```python
from build123d import *

# Parameters (mm, degrees)
ESBO_O1_R                = 12.5
RESSALTO_EXTRUS_O1_DEPTH = 30
ESBO_O2_R                = 8
CORTE_EXTRUS_O1_DEPTH    = 15
ESBO_O3_W                = 3
ESBO_O3_H                = 5
CORTE_EXTRUS_O2_DEPTH    = 6.5


with BuildPart() as part:
    # Esboço1 → Ressalto-extrusão1 (new body)
    with BuildSketch(Plane(origin=(0, 0, 0), x_dir=(1, 0, 0), z_dir=(0, 1, 0))):
        with Locations(Location((0, 0, 0), (0, 0, 270))):
            Circle(ESBO_O1_R)
    extrude(amount=RESSALTO_EXTRUS_O1_DEPTH)

    # Esboço2 → Corte-extrusão1 (cut)
    with BuildSketch(Plane(origin=(0, 30, 0), x_dir=(1, 0, 0), z_dir=(0, 1, 0))):
        with Locations(Location((0, 0, 0), (0, 0, 270))):
            Circle(ESBO_O2_R)
    extrude(amount=-CORTE_EXTRUS_O1_DEPTH, mode=Mode.SUBTRACT)

    # Esboço3 → Corte-extrusão2 (cut)
    with BuildSketch(Plane.XZ):
        Rectangle(ESBO_O3_W, ESBO_O3_H)
    extrude(amount=-CORTE_EXTRUS_O2_DEPTH, mode=Mode.SUBTRACT)


solid = part.part
```
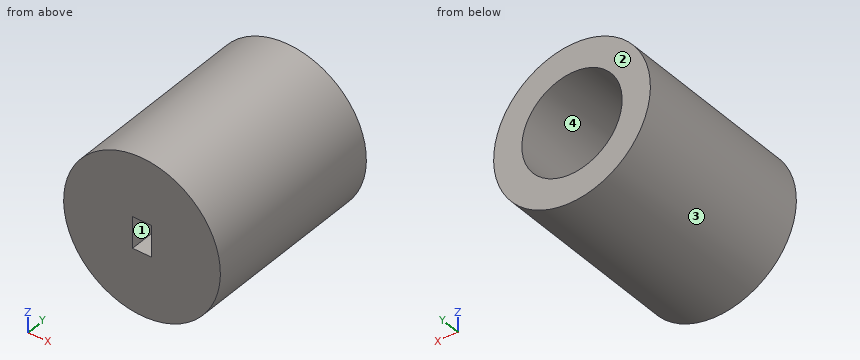
Here's how the part is built. I have some questions about the finished solid (model axes, mm). Face numbers are marked on the shaded views. Coordinates: 2 decimals unless noted, no trailing zeros. Order: outer loops, then holes, each group sorted by start corner. A loop starts at its lowest first (then second) coordinate and runs counter-clockwise, first axis right, second up.
Item 1: I'm going to push flat-ended pins straight in: pin 1 Ø1.5 at (y, z) = (3.5, -1) entering from +X; pin 2 Ø8 at (x, z) = (1, -3) entering from +Y; pin 3 Ø2.5 at (x, z) = (0, 0.5) entering from -Y. Where does each tip first touch, or does it pass through?
Response values:
pin 1: stops at x = 12.5
pin 2: stops at y = 15
pin 3: stops at y = 6.5
Item 2: If we section it at D-D, the plane y = 18.75: List the corners of the cut face in (x, z) for me.
Response values:
outline: circle Ø25 at (0, 0); hole circle Ø16 at (0, 0)
Item 3: If we section it at C-C, the plane x = 0: List the corners of the cut face in (y, z) for me, then the cut area to 4 significant figures.
Response values:
outline: (0, -12.5) - (30, -12.5) - (30, -8) - (15, -8) - (15, 8) - (30, 8) - (30, 12.5) - (0, 12.5) - (0, 2.5) - (6.5, 2.5) - (6.5, -2.5) - (0, -2.5) - close
area: 477.5 mm2
Item 4: Thinking about a two-plate mould opening in Z: for the marked faces 1, 2, 3 and 4, which applies, pulls with the +Z half, pulls with the -Z half, needs draft (parallel to the pull), parting line crosses it, or undercut?
Response values:
face 1: undercut
face 2: needs draft
face 3: parting line crosses it
face 4: undercut
Item 5: I need wall thicknesses on probe 1 along X at (y, z) = (19.25, 0); probe 2 along Y at (x, z) = (2.5, 1.25); probe 3 along X at (y, z) = (19.25, 7.25). Which ranges of each line are inside material? Lowest first, please.
Response values:
probe 1: x = -12.5 to -8, 8 to 12.5
probe 2: y = 0 to 15
probe 3: x = -10.18 to -3.38, 3.38 to 10.18
Item 6: If we section it at A-A, the plane y = 3.5: List the corners of the cut face in (x, z) for me, then the cut area to 3 significant figures.
Response values:
outline: circle Ø25 at (0, 0); hole (-1.5, -2.5) - (1.5, -2.5) - (1.5, 2.5) - (-1.5, 2.5) - close
area: 476 mm2
Item 7: If we section it at B-B, the plane z = 0: List the corners of the cut face in (x, y) for me, then the cut area to 4 significant figures.
Response values:
outline: (-12.5, 0) - (-1.5, 0) - (-1.5, 6.5) - (1.5, 6.5) - (1.5, 0) - (12.5, 0) - (12.5, 30) - (8, 30) - (8, 15) - (-8, 15) - (-8, 30) - (-12.5, 30) - close
area: 490.5 mm2
